Source: CAD feature listing. Evaluate the final solid. Frame: model axes, mm. Give positions to 0.01 mm unless a question says otherwise; leave off trailing zeros. Put each result on its own line as item: value.
Autodesk Inventor part; units mm, degrees
ref_plane "YZ Plane" through (0, 0, 0) normal (1, 0, 0) x (0, 1, 0)
ref_plane "XZ Plane" through (0, 0, 0) normal (0, 1, 0) x (-1, 0, 0)
ref_plane "XY Plane" through (0, 0, 0) normal (0, 0, 1) x (1, 0, 0)
sketch "Skizze1" plane through (0, 0, 0) normal (0, 1, 0) x (-1, 0, 0)
  line L0 (0, 0) -> (35, 0)
  line L1 (35, 0) -> (35, 6)
  line L2 (35, 6) -> (29, 6)
  line L3 (0, 25) -> (0, 0)
  arc A0 (29, 6) -> (0, 25) centre (-0.2408, -6.9991) ccw
  dimension "d0" = 35
  dimension "d1" = 12
  dimension "d2" = 6
  dimension "d5" = 50
  dimension "d6" = 32
revolve "Umdrehung1" add sketch "Skizze1" angle 360 about axis through (0, 0, 0) along (-1, 0, 0)
sketch "Skizze3" plane through (-35, 0, 0) normal (-1, 0, 0) x (0, 0, 1)
  circle A0 centre (0, 0) radius 6
hole "Bohrung2" at (-35, 0, 0) direction (1, 0, 0) diameter 6.647 depth 6
fillet "Rundung1" radius 2 1 edges at (-29, 0, -6)
sketch "Skizze5" plane through (0, 0, 0) normal (0, 1, 0) x (-1, 0, 0)
  arc A0 (0, -25) -> (28.4771, -7.1177) centre (-0.2408, 6.9991) ccw
  arc A1 (28.4771, 7.1177) -> (0, 25) centre (-0.2408, -6.9991) ccw
  line L0 (0, 0) -> (39.0917, 0)
  arc A2 (1, -24.4765) -> (28.0284, -6.8971) centre (-0.2408, 6.9991) ccw
  line L1 (1, -24.4765) -> (1, 0)
  line L2 (35, -6) -> (35, 6)
  line L3 (30.272, 6) -> (30.272, -6)
  line L4 (29, -3.3235) -> (35, -3.3235)
  arc A3 (30.272, -6) -> (28.4771, -7.1177) centre (30.272, -8) ccw
  line L5 (29, -3.3235) -> (29, 3.3235)
  arc A4 (28.0284, -6.8971) -> (29, -3.3235) centre (-11.0986, 5.66) ccw
  point P0 (29, 0)
  dimension "d25" = 1
  dimension "d26" = 0.5
revolve "Umdrehung2" cut sketch "Skizze5" angle 360 about axis through (0, 0, 0) along (-1, 0, 0) contours L0 L5 A4 A2 L1
sketch "Skizze6" plane through (0, 0, 0) normal (1, 0, 0) x (0, 0, -1)
  circle A0 centre (0, 0) radius 25
hole "Bohrung3" at (0, 0, 0) direction (-1, 0, 0) diameter 50 depth 1
properties part number "BRS_cover" material "Blei"
(1) Draft query along Z for faces 1 (the cylindrical face through (-33, 0, -6)), 2 (the flat face through (-1, 17, -18)), 3 (the cylindrical face through (-31.96, 1.27, 3.07)). Return one class per face: released by +Z, released by -Z, zero draft, split by the parting line, or undercut.
Calculated:
face 1: split by the parting line
face 2: zero draft
face 3: undercut
(2) Line query: probe 1 along Z at (x, y) = (-33, 0); probe 2 along Z at (x, y) = (-13.5, -11). Output: solid intervals per line, ascending. Write a range as from..to.
Calculated:
probe 1: z = -6..-3.32, 3.32..6
probe 2: z = -18.94..-18.29, 18.29..18.94
(3) First-contact query: P1, Ø1.5, axis at x = -14, y = 10.5, coming from the +Z side; P2, Ø2, axis at x = -7.5, y = -12, coming from the +Z side; P3, Ø8, axis at x = -24.5, y = 3, coming from the -Z side; P4, Ø5.5, axis at y = 0, z = 0, coming from the -X side. Flat tips, straight axial feed; report the tip coordinate or a pass-through.
Calculated:
P1: stops at z = 19.52
P2: stops at z = 21.45
P3: stops at z = -17.16
P4: passes through
